Build history of the part. All positions in model axes, mm. Face numbers are marked on the shaded views. Coordinates: 2 decimals unless noted, no trailing zeros. Write each loop counter-clockwise with the first axis right and the second up, starting at its lowest first coordinate (ties: lowest second). Pieces come first, ordered by that corner, then holes.
from build123d import *

# Parameters (mm, degrees)
BOSS_EXTRUDE1_DEPTH      = 1.45
BOSS_EXTRUDE1_DEPTH_BACK = 1.45
SKETCH3_W                = 13
SKETCH3_H                = 3
SKETCH3_R                = 0.5
SKETCH4_R                = 5
CUT_EXTRUDE1_DEPTH       = 20
FILLET1_R                = 2


with BuildPart() as part:
    # Sketch1 → Revolve1 (revolve)
    with BuildSketch(Plane.XY, mode=Mode.PRIVATE) as revolve1_sk:
        with BuildLine():
            Line((-8.5, 0), (-8.5, 25))
            add(Edge.make_bspline(
                [(-8.5, 25), (-8.597015347, 26.01504006), (-8.907000797, 27.967323593), (-10.203463046, 30.716511268), (-11.74686042, 33.10560974), (-13.777222786, 35.500816023), (-16.044814471, 36.474123076), (-17.015460227, 34.847167716)],
                knots=[0, 0, 0, 0, 0.199432853, 0.381102799, 0.589074274, 0.751073338, 1, 1, 1, 1], degree=3))
            add(Edge.make_bspline(
                [(-17.015460227, 34.847167716), (-15.061693604, 34.149149549), (-12.546917313, 30.799465382), (-10.772360994, 27.13941137), (-10.5, 25)],
                knots=[0, 0, 0, 0, 0.483303416, 1, 1, 1, 1], degree=3))
            Line((-10.5, 25), (-10.5, 0))
            Line((-10.5, 0), (-8.5, 0))
        make_face()
    revolve(revolve1_sk.sketch.rotate(Axis((0, 0, 0), (0, 1, 0)), 270), axis=Axis((0, 0, 0), (0, 1, 0)))

    # Sketch3 → Boss-Extrude1 (add, two sides: drawn at the far end of the back side and taken through both)
    with BuildSketch(Plane.XY.offset(-BOSS_EXTRUDE1_DEPTH_BACK)):
        with Locations((4, 1.5)):
            Rectangle(SKETCH3_W, SKETCH3_H)
        with Locations((0, 1.5)):
            Circle(SKETCH3_R, mode=Mode.SUBTRACT)
    extrude(amount=BOSS_EXTRUDE1_DEPTH + BOSS_EXTRUDE1_DEPTH_BACK)

    # Sketch4 → Cut-Extrude1 (cut)
    with BuildSketch(Plane.XY.offset(1.45)):
        Circle(SKETCH4_R)
    extrude(amount=CUT_EXTRUDE1_DEPTH, mode=Mode.SUBTRACT)

    # Fillet1
    # the kernel refuses this fillet: 2 mm, written as the material it takes off along each edge
    with BuildSketch(Plane(origin=(13.375410438, 3, -1.45), x_dir=(0, 0, 1), z_dir=(-1, 0, 0))) as fillet1_piece_1_section:
        with BuildLine():
            CenterArc((FILLET1_R, -FILLET1_R), FILLET1_R, 90, 90)
            Line((0, -FILLET1_R), (0, 0))
            Line((0, 0), (FILLET1_R, 0))
        make_face()
    fillet1_piece_1 = extrude(amount=20.875410438, mode=Mode.PRIVATE)
    fillet1_piece_1 = fillet1_piece_1 & Plane(origin=(0, 2.559869682, 0), x_dir=(0, 0, -1), z_dir=(0, 1, 0)) * Cylinder(8.5, 50, mode=Mode.PRIVATE)
    add(fillet1_piece_1, mode=Mode.SUBTRACT)
    with BuildSketch(Plane(origin=(-7.5, 3, 1.45), x_dir=(0, -1, 0), z_dir=(1, 0, 0))) as fillet1_piece_2_section:
        with BuildLine():
            CenterArc((FILLET1_R, FILLET1_R), FILLET1_R, 180, 90)
            Line((0, FILLET1_R), (0, 0))
            Line((0, 0), (FILLET1_R, 0))
        make_face()
    fillet1_piece_2 = extrude(amount=20.875410438, mode=Mode.PRIVATE)
    fillet1_piece_2 = fillet1_piece_2 & Plane(origin=(0, 2.559861322, 0), x_dir=(0, 0, -1), z_dir=(0, 1, 0)) * Cylinder(8.5, 50, mode=Mode.PRIVATE)
    add(fillet1_piece_2, mode=Mode.SUBTRACT)


solid = part.part
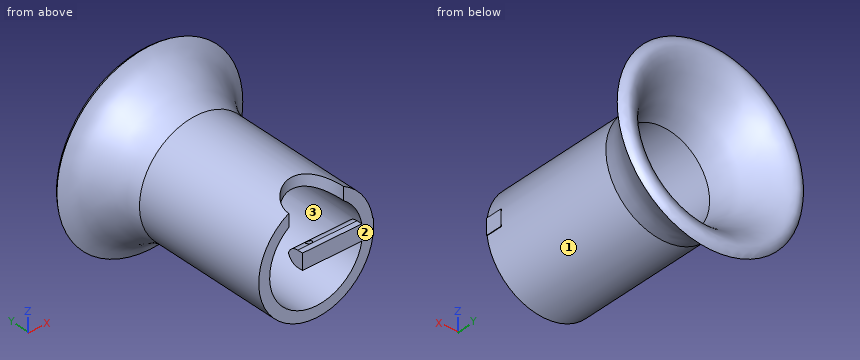
(1) Probe L1, parallel to X at y = 1.5, z = 0.1; L2, parallel to X at y = 15.25, z = 0; L3, parallel to X at y = 13, z = -6. List the from-to ranges inside material, lowest first.
(2) Slice it at A-A, the plane y = 1.5. List the corners of the cut face in (x, z), and give its area (3 significant figures).
(3) Slice it at B-B, the plane x = 4. Give the number of separate pieces and of enclosed holes in the cut face, and give its area (3 significant figures).
(4) Two-plate mould, pull along X, no slides. Class the marked faces 1, 2 and 3: pulls with the +X half, pulls with the -X half, needs draft (parallel to the pull), parting line crosses it, or undercut.
(5) Flat gauge pins, fed straight in: P1, Ø10, axis at x = 0.5, y = 11, coming from the -Z side; P2, Ø10, axis at x = 0, z = 0, coming from the +Y side; P3, Ø2.5, axis at y = 1.5, z = 0, coming from the -X side; P4, Ø2, axis at y = 13.5, z = -12.5, coming from the -X side. Where does each tip first touch, or does it go through?
(6) Slice it at C-C, the plane y = 24. List the corners of the cut face in (x, z), and give its area (3 significant figures).
Results:
1. L1: x = -10.5 to -8.5, -2.5 to -0.5, 0.5 to 10.5
1. L2: x = -10.5 to -8.5, 8.5 to 10.5
1. L3: x = -8.62 to -6.02, 6.02 to 8.62
2. outline: (-4.77, 7.04) - (-4.77, 9.35) arc R10.5 ccw (long way) to (10.4, -1.45) - (10.5, -1.45) - (10.5, 1.45) - (10.4, 1.45) arc R10.5 ccw to (4.77, 9.35) - (4.77, 7.04) arc R8.5 cw to (8.39, 1.39) - (0.5, 1.39) - (0.5, -1.39) - (8.39, -1.39) arc R8.5 cw (long way) to start; (-2.5, -1.39) - (-0.5, -1.39) - (-0.5, 1.39) - (-2.5, 1.39) - close
2. area: 127 mm2
3. separate pieces: 3
3. enclosed holes: 0
3. area: 167 mm2
4. face 1: parting line crosses it
4. face 2: needs draft
4. face 3: undercut
5. P1: stops at z = -10.5
5. P2: stops at y = 2.92
5. P3: stops at x = -10.5
5. P4: passes through
6. outline: circle Ø21 at (0, 0); hole circle Ø17 at (0, 0)
6. area: 119 mm2
